Study the drawing (mm; zero at the part's minimum x, y, z) and answer. A direction names the side the tool comes from. Coordinates: 2 decimals unless noted, no trailing zeros. Loops run counter-clockwise (first coordinate to the right, second up) from the corner with the lowest first, then second, coordinate; pieces in that order, holes last. Notation, with made-up numbers: (35, 58.25) -> (54, 58.25) arc R20 cw to (54, 70.25) -> close; hole circle Ø9 at (75.25, -31.5). An arc over 180 degrees is marked (long way). Answer in a Markdown table with one row per item.
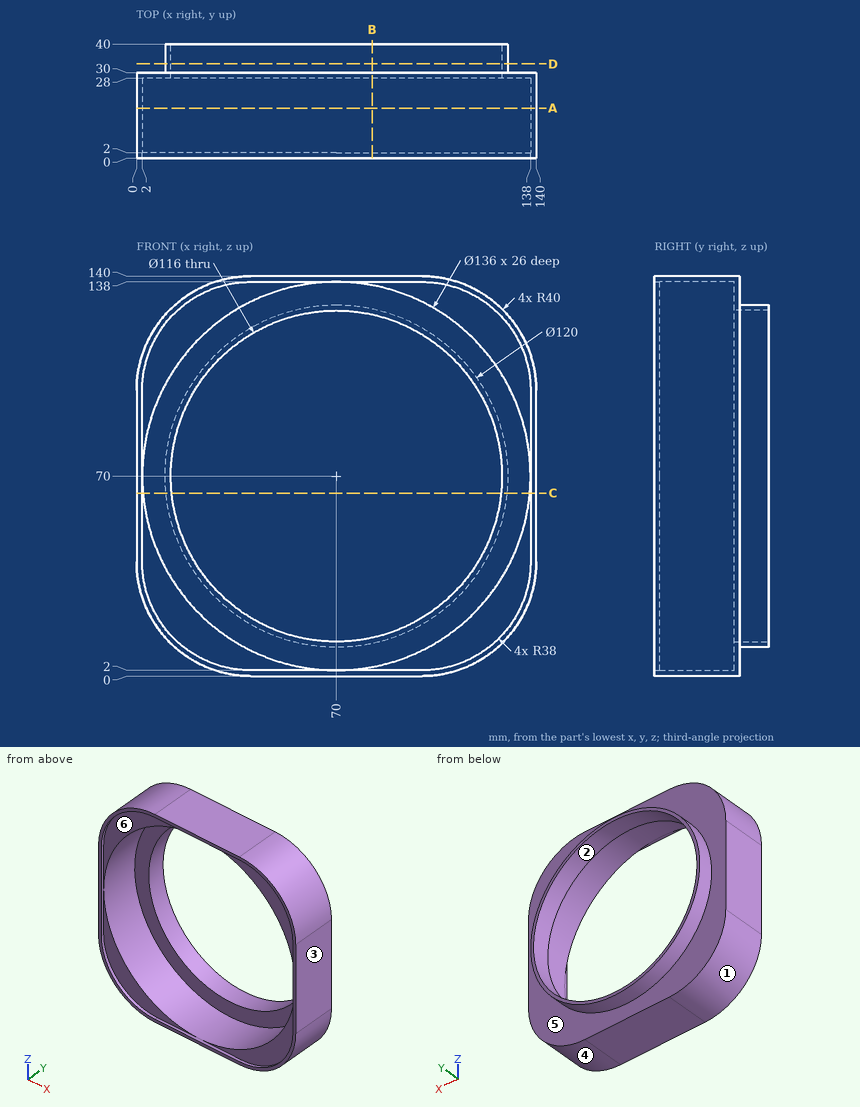
1. Given pin 1 Ø3 at (x, y) = (105, 5.5) entering from -Z; pin 2 Ø1.5 at (x, z) = (19.5, 121) entering from +Y; pin 3 Ø1 at (x, y) = (29.5, 32) entering from -Z, each flat-ended and moving along its own axis, determine where each tip first touches the part or whether it passes through.
A:
| item | result |
|---|---|
| pin 1 | stops at z = 0.15 |
| pin 2 | stops at y = 30 |
| pin 3 | stops at z = 25.28 |
2. A cutting plane is placed at D-D on y = 33. Give the vertices of the cut face in (x, z).
A:
| item | result |
|---|---|
| outline | circle Ø120 at (70, 70); hole circle Ø116 at (70, 70) |
3. A cutting plane is placed at C-C on z = 64. Give the vertices of the cut face in (x, y).
A:
| item | result |
|---|---|
| outline | (0, 0) -> (2, 0) -> (2, 2) -> (2.27, 2) -> (2.27, 28) -> (12.31, 28) -> (12.31, 40) -> (10.3, 40) -> (10.3, 30) -> (0, 30) -> close; (127.69, 28) -> (137.73, 28) -> (137.73, 2) -> (138, 2) -> (138, 0) -> (140, 0) -> (140, 30) -> (129.7, 30) -> (129.7, 40) -> (127.69, 40) -> close |
4. A tool of negligible diameter and unlimited length cuts with its end or side. For the marked faces 4, 5 and 6, from which of +Z, -Z, +X, -X, +Y, -Y can it reach the whole face along a straight path? Write none if from no direction.
A:
| item | result |
|---|---|
| face 4 | -Z, +X, +Y, -Y |
| face 5 | +Y |
| face 6 | -Y |
5. Find the intervals of material crossed by probe 1 along X at (y, z) = (3.5, 70); probe 2 along X at (y, z) = (37.5, 70), in increasing order.
A:
| item | result |
|---|---|
| probe 1 | x = 0 to 2, 138 to 140 |
| probe 2 | x = 10 to 12, 128 to 130 |
6. A cutting plane is placed at A-A on y = 17.5. Give the vertices of the cut face in (x, z), and give its area (3 significant figures).
A:
| item | result |
|---|---|
| outline | (0, 40) arc R40 ccw to (40, 0) -> (100, 0) arc R40 ccw to (140, 40) -> (140, 100) arc R40 ccw to (100, 140) -> (40, 140) arc R40 ccw to (0, 100) -> close; hole circle Ø136 at (70, 70) |
| area | 3,700 mm2 |
7. A cutting plane is placed at B-B on x = 82.5. Give the vertices of the cut face in (y, z), and give its area (3 significant figures).
A:
| item | result |
|---|---|
| outline | (0, 0) -> (30, 0) -> (30, 11.32) -> (40, 11.32) -> (40, 13.36) -> (28, 13.36) -> (28, 3.16) -> (2, 3.16) -> (2, 2) -> (0, 2) -> close; (0, 138) -> (2, 138) -> (2, 136.84) -> (28, 136.84) -> (28, 126.64) -> (40, 126.64) -> (40, 128.68) -> (30, 128.68) -> (30, 140) -> (0, 140) -> close |
| area | 267 mm2 |
8. The mould has two halves that part along X. Classify the marked faces 1, 2 and 3: pulls with the +X half, pulls with the -X half, needs draft (parallel to the pull), parting line crosses it, or undercut.
A:
| item | result |
|---|---|
| face 1 | pulls with the -X half |
| face 2 | undercut |
| face 3 | pulls with the +X half |
